```python
from build123d import *

# Parameters (mm, degrees)
MODEL_R         = 11
MODEL_R_2       = 9.5
MODEL_R_3       = 1.5
MODEL_R_4       = 3
EXTRUDE_1_DEPTH = 3


with BuildPart() as part:
    # Model → 凸台-拉伸1 (new body)
    with BuildSketch(Plane.XY):
        with BuildLine():
            Line((1088.508697922, 149.67262706), (1083.05209603, 180.618554166))
            ThreePointArc((1083.05209603, 180.618554166), (1077.92179388, 189.504498148), (1068.279979735, 193.013831501))
            Line((1068.279979735, 193.013831501), (1051.677026847, 193.013831501))
            ThreePointArc((1051.677026847, 193.013831501), (1043.967976827, 190.481426631), (1039.262378471, 183.870838854))
            Line((1039.262378471, 183.870838854), (1004.158643075, 70.881546432))
            ThreePointArc((1004.158643075, 70.881546432), (1029.249360335, 21.222627878), (1079.700778213, 44.67911352))
            Line((1079.700778213, 44.67911352), (1084.260160223, 56.556709735))
            ThreePointArc((1084.260160223, 56.556709735), (1097.111256858, 72.858248103), (1116.93547515, 79.013831501))
            Line((1116.93547515, 79.013831501), (1288.003781731, 79.013831501))
            ThreePointArc((1288.003781731, 79.013831501), (1308.078957003, 72.684153051), (1320.893023458, 55.984536518))
            Line((1320.893023458, 55.984536518), (1324.769856321, 45.333025768))
            ThreePointArc((1324.769856321, 45.333025768), (1372.710322957, 20.37679845), (1401.749871273, 65.959758608))
            Line((1401.749871273, 65.959758608), (1401.710502358, 66.183030822))
            ThreePointArc((1401.710502358, 66.183030822), (1405.023616532, 81.127523103), (1417.933693865, 89.352149436))
            Line((1417.933693865, 89.352149436), (1425.704857508, 90.722415258))
            ThreePointArc((1425.704857508, 90.722415258), (1426.889650039, 91.406455544), (1427.357561153, 92.692030764))
            Line((1427.357561153, 92.692030764), (1427.357561153, 99.013831501))
            ThreePointArc((1427.357561153, 99.013831501), (1418.570764588, 120.227034937), (1397.357561153, 129.013831501))
            Line((1397.357561153, 129.013831501), (1113.128891747, 129.013831501))
            ThreePointArc((1113.128891747, 129.013831501), (1097.059201505, 134.862720423), (1088.508697922, 149.67262706))
        make_face()
        with Locations((1362.357561153, 59.013831501)):
            Circle(MODEL_R, mode=Mode.SUBTRACT)
        with Locations((1042.357561153, 59.013831501)):
            Circle(MODEL_R, mode=Mode.SUBTRACT)
        with Locations((1062.357561153, 154.013831501)):
            Circle(MODEL_R_2, mode=Mode.SUBTRACT)
        with Locations((1151.357561153, 91.513831501)):
            Circle(MODEL_R_3, mode=Mode.SUBTRACT)
        with Locations((1163.357561153, 91.513831501)):
            Circle(MODEL_R_3, mode=Mode.SUBTRACT)
        with Locations((1271.357561153, 91.513831501)):
            Circle(MODEL_R_3, mode=Mode.SUBTRACT)
        with Locations((1283.357561153, 91.513831501)):
            Circle(MODEL_R_3, mode=Mode.SUBTRACT)
        with Locations((1391.357561153, 91.513831501)):
            Circle(MODEL_R_3, mode=Mode.SUBTRACT)
        with Locations((1403.357561153, 91.513831501)):
            Circle(MODEL_R_3, mode=Mode.SUBTRACT)
        with Locations((1093.357561153, 114.513831501)):
            Circle(MODEL_R_3, mode=Mode.SUBTRACT)
        with Locations((1081.357561153, 114.513831501)):
            Circle(MODEL_R_3, mode=Mode.SUBTRACT)
        with Locations((1046.357561153, 94.513831501)):
            Circle(MODEL_R_3, mode=Mode.SUBTRACT)
        with Locations((1058.357561153, 94.513831501)):
            Circle(MODEL_R_3, mode=Mode.SUBTRACT)
        with Locations((1071.357561153, 70.513831501)):
            Circle(MODEL_R_3, mode=Mode.SUBTRACT)
        with Locations((1083.357561153, 70.513831501)):
            Circle(MODEL_R_3, mode=Mode.SUBTRACT)
        with Locations((1036.357561153, 34.513831501)):
            Circle(MODEL_R_3, mode=Mode.SUBTRACT)
        with Locations((1048.357561153, 34.513831501)):
            Circle(MODEL_R_3, mode=Mode.SUBTRACT)
        with Locations((1356.357561153, 34.513831501)):
            Circle(MODEL_R_3, mode=Mode.SUBTRACT)
        with Locations((1368.357561153, 34.513831501)):
            Circle(MODEL_R_3, mode=Mode.SUBTRACT)
        with Locations((1062.357561153, 172.013831501)):
            Circle(MODEL_R_3, mode=Mode.SUBTRACT)
        with Locations((1080.357561153, 154.013831501)):
            Circle(MODEL_R_3, mode=Mode.SUBTRACT)
        with Locations((1062.357561153, 136.013831501)):
            Circle(MODEL_R_3, mode=Mode.SUBTRACT)
        with Locations((1044.357561153, 154.013831501)):
            Circle(MODEL_R_3, mode=Mode.SUBTRACT)
        with Locations((1042.380322879, 130.30919164)):
            Circle(MODEL_R_3, mode=Mode.SUBTRACT)
        with Locations((1032.316276064, 123.77352322)):
            Circle(MODEL_R_3, mode=Mode.SUBTRACT)
        with Locations((1042.357561153, 73.013831501)):
            Circle(MODEL_R_3, mode=Mode.SUBTRACT)
        with Locations((1056.357561153, 59.013831501)):
            Circle(MODEL_R_3, mode=Mode.SUBTRACT)
        with Locations((1042.357561153, 45.013831501)):
            Circle(MODEL_R_3, mode=Mode.SUBTRACT)
        with Locations((1028.357561153, 59.013831501)):
            Circle(MODEL_R_3, mode=Mode.SUBTRACT)
        with Locations((1362.357561153, 73.013831501)):
            Circle(MODEL_R_3, mode=Mode.SUBTRACT)
        with Locations((1376.357561153, 59.013831501)):
            Circle(MODEL_R_3, mode=Mode.SUBTRACT)
        with Locations((1362.357561153, 45.013831501)):
            Circle(MODEL_R_3, mode=Mode.SUBTRACT)
        with Locations((1348.357561153, 59.013831501)):
            Circle(MODEL_R_3, mode=Mode.SUBTRACT)
        with Locations((1257.357561153, 88.013831501)):
            Circle(MODEL_R_4, mode=Mode.SUBTRACT)
        with Locations((1043.885858479, 181.699972429)):
            Circle(MODEL_R_3, mode=Mode.SUBTRACT)
        with Locations((1052.99702044, 173.890572471)):
            Circle(MODEL_R_3, mode=Mode.SUBTRACT)
    extrude(amount=EXTRUDE_1_DEPTH)


solid = part.part
```
Design review of the part built by this model. Coordinates are the model's own, in mm. A direction names the side the tool comes from. Coordinates: 2 decimals unless noted, no trailing zeros. Loops run counter-clockwise (first coordinate to the right, second up) from the corner with the lowest first, then second, coordinate; pieces in that order, holes last. Notation, with made-up numbers: (12, -30) - (71, -30) arc R23 cw to (71, -19) - close; hole circle Ø6 at (-29, 73). An arc over 180 degrees is marked (long way). Use CSV: the item, a comma, the result in double quotes. Start each with the question number.
1) Consider section B-B on x = 1293.5. Write out the cut boundary in (y, z).
2) For pin 1 Ø1 at (x, z) = (1056.5, 0.5) entering from -Y, flat-tipped, find the tip position at first contact; note if it passes through.
3) Consider section A-A on z = 1.5. Give the number of separate pieces and of enclosed holes in the cut face, then the cut area to 3 significant figures.
4) The part is to be moulded in two halves that separate along Y. For faces 3 (the cylindrical face through (1044.06, 190.55, 1.48)), 4 (the flat face through (1212, 107, 0)), 5 (the cylindrical face through (1404.9, 80.95, 1.48)), 6 (the cylindrical face through (1307.833, 72.855, 1.479)), say which applies: +Y half, -Y half, draft (parallel to the pull), parting line (faces both ways), or undercut.
5) Consider section C-C on y = 106. Write out the cut boundary in (x, z).
6) Wall thickness on L1, parallel to Y at x = 1047, z = 1.05; L2, parallel to X at y = 44.5, z = 1.4; L3, parallel to X at y = 54, z = 0.25: over which ranges is each line inside the solid? List them lowest first. Write a range as from..to.
7) Tool access review of faces 1 (the cylindrical face through (1096.87, 72.69, 1.48)), 2 (the cylindrical face through (1078.034, 189.41, 1.479)): name each direction out of +Z, -Z, +X, -X, +Y, -Y from which nothing blocks a thin tool from reaching the whole face with its end or side.
Geometry says:
1,outline,"(78.58, 0) - (129.01, 0) - (129.01, 3) - (78.58, 3) - close"
2,pin 1,"y = 21.41"
3,separate pieces,"1"
3,enclosed holes,"36"
3,area,"31,200 mm^2"
4,face 3,"+Y half"
4,face 4,"draft"
4,face 5,"undercut"
4,face 6,"-Y half"
5,outline,"(1015.07, 0) - (1426.53, 0) - (1426.53, 3) - (1015.07, 3) - close"
6,L1,"19.28..33.88, 35.15..49.04, 68.99..93.16, 95.87..192.14"
6,L2,"1005.08..1040.95, 1043.77..1079.63, 1325.08..1360.95, 1363.77..1399.63"
6,L3,"1002.67..1032.57, 1052.15..1083.28, 1321.62..1352.57, 1372.15..1402.04"
7,face 1,"+Z, -Z, -Y"
7,face 2,"+Z, -Z, +X, +Y"
